For this review, take the finished solid that the model builds, in its own axes (mm). A direction names the side the tool comes from. Coordinates: 2 decimals unless noted, no trailing zeros. Write each loop counter-clockwise with the first axis right and the second up, starting at its lowest first coordinate (ties: lowest second). Pieces come first, ordered by that corner, then holes. Notation, with made-up numbers: (80.5, 22.25) -> (137.5, 22.25) arc R17 ccw to (137.5, 50.25) -> close; hole circle Ø4 at (-4.75, 87.25). An arc over 180 degrees is marked (long way). Put each result on its own line as item: value. Start each with the question number.
Item 1: To check wall thickness, follow L1, parallel to Y at x = 9, z = 0.15; L2, parallel to Y at x = -26.5, z = -1.75; L3, parallel to Y at x = 33, z = -1.2. State the ranges of each line that lie inside material, in increasing order.
Item 2: Consider section D-D on z = 0.15. Give the number of separate pieces and of enclosed holes in the cut face, and give its area (3 significant figures).
Item 3: Consider section B-B on x = 1. Give the boundary of the cut face in (y, z), and give its area (3 significant figures).
Item 4: Consider section C-C on y = 15. Give the boundary of the cut face in (x, z), and give its area (3 significant figures).
Item 5: For faces 4 (the flat face through (-20.334, -33.421, -1.44)), 5 (the flat face through (-35.9, 0, -2)), 6 (the flat face through (-7, 38, -0.7)), 7 (the flat face through (4.01, -24.66, 0.04)), 8 (the flat face through (35.9, 0, -2)), list the 3-axis set-ups (+Z, -Z, +X, -X, +Y, -Y) from which the entire face can be reached by the end or side of a thin tool; tool diameter is ignored.
Item 6: Consider section A-A on y = -7.5. Give the boundary of the cut face in (x, z).
Item 7: Insertion check: P1, Ø8, axis at x = 28, y = 39, coming from the -Z side; P2, Ø1.5, axis at y = -36.5, z = -1.5, coming from the +X side; P3, Ø1.1, axis at y = -6, z = -1.5, coming from the -X side. Each pin has a flat end and moves straight along its axis. Give the tip position at first contact, or say it passes through.
Item 8: The part is to be moulded in two halves that separate along Y. For faces 1 (the flat face through (20.7, -33.88, -1.44)), 2 (the flat face through (-1, 12, 0.8)), 3 (the flat face through (33.4, 14.8, -1.7)), say which applies: +Y half, -Y half, draft (parallel to the pull), parting line (faces both ways), or undercut.
```python
from build123d import *

# Parameters (mm, degrees)
ESBO_O2_W                = 80
ESBO_O2_H                = 100
ESBO_O2_W_2              = 55.6
ESBO_O2_H_2              = 18.4
RESSALTO_EXTRUS_O1_DEPTH = 0.8
RESSALTO_EXTRUS_O2_DEPTH = 2.2
CHANFRO3_SIZE            = 5
ESBO_O5_W                = 10
ESBO_O5_H                = 20
CORTE_EXTRUS_O1_DEPTH    = 10
CHANFRO4_SIZE            = 2
CHANFRO5_SIZE            = 2
RESSALTO_EXTRUS_O3_DEPTH = 0.7
ESBO_O7_W                = 61.8
ESBO_O7_H                = 24.6
ESBO_O7_W_2              = 55.6
ESBO_O7_H_2              = 18.4
RESSALTO_EXTRUS_O4_DEPTH = 2
ESBO_O8_W                = 61.8
ESBO_O8_H                = 24.6
RESSALTO_EXTRUS_O5_DEPTH = 0.6
CHANFRO6_SIZE            = 5
ESBO_O11_W               = 55.6
ESBO_O11_H               = 18.4
CORTE_EXTRUS_O2_DEPTH    = 0.9


with BuildPart() as part:
    # Esboço2 → Ressalto-extrusão1 (new body)
    with BuildSketch(Plane.XY):
        Rectangle(ESBO_O2_W, ESBO_O2_H)
        Rectangle(ESBO_O2_W_2, ESBO_O2_H_2, mode=Mode.SUBTRACT)
    extrude(amount=RESSALTO_EXTRUS_O1_DEPTH)

    # Esboço4 → Ressalto-extrusão2 (add)
    with BuildSketch(Plane(origin=(0, 0, 0), x_dir=(-1, 0, 0), z_dir=(0, 0, -1))):
        Polygon((40, -41.996094703), (20.243124237, -17.3), (35.9, -17.3), (35.9, 17.3), (20.243124237, 17.3), (40, 41.996094703), (40, 50), (33.596875763, 50), (7.436875763, 17.3), (-7.436875763, 17.3), (-33.596875763, 50), (-40, 50), (-40, 41.996094703), (-20.243124237, 17.3), (-35.9, 17.3), (-35.9, -17.3), (-20.243124237, -17.3), (-40, -41.996094703), (-40, -50), (-33.596875763, -50), (-7.436875763, -17.3), (7.436875763, -17.3), (33.596875763, -50), (40, -50), align=None)
        Polygon((3.436875763, 12.3), (5, 12.3), (16.243124237, 12.3), (30.9, 12.3), (30.9, -12.3), (16.243124237, -12.3), (5, -12.3), (3.436875763, -12.3), (-3.436875763, -12.3), (-5, -12.3), (-16.243124237, -12.3), (-30.9, -12.3), (-30.9, 12.3), (-16.243124237, 12.3), (-5, 12.3), (-2.810379517, 12.3), align=None, mode=Mode.SUBTRACT)
    extrude(amount=RESSALTO_EXTRUS_O2_DEPTH)

    # Chanfro3
    chanfro3_edges = [part.edges().sort_by_distance(p)[0] for p in [
        (-35.9, 17.3, -1.1),
        (35.9, 17.3, -1.1),
        (35.9, -17.3, -1.1),
        (-35.9, -17.3, -1.1),
    ]]
    chamfer(chanfro3_edges, length=CHANFRO3_SIZE)

    # Esboço5 → Corte-extrusão1 (cut)
    with BuildSketch(Plane(origin=(0, 0, 0), x_dir=(-1, 0, 0), z_dir=(0, 0, -1))):
        with Locations((0, 33.65)):
            Rectangle(ESBO_O5_W, ESBO_O5_H)
        with Locations((0, -33.65)):
            Rectangle(ESBO_O5_W, ESBO_O5_H)
    extrude(amount=-CORTE_EXTRUS_O1_DEPTH, mode=Mode.SUBTRACT)

    # Chanfro4
    chanfro4_edges = [part.edges().sort_by_distance(p)[0] for p in [
        (-5, 43.65, 0.4),
        (-5, 23.65, 0.4),
        (5, 23.65, 0.4),
        (5, 43.65, 0.4),
        (-5, -23.65, 0.4),
        (-5, -43.65, 0.4),
        (5, -43.65, 0.4),
        (5, -23.65, 0.4),
    ]]
    chamfer(chanfro4_edges, length=CHANFRO4_SIZE)

    # Chanfro5
    chanfro5_edges = [part.edges().sort_by_distance(p)[0] for p in [
        (-40, 50, -0.7),
        (40, 50, -0.7),
        (40, -50, -0.7),
        (-40, -50, -0.7),
    ]]
    chamfer(chanfro5_edges, length=CHANFRO5_SIZE)

    # Esboço6 → Ressalto-extrusão3 (add)
    # profile 1 of 4: a face of its own
    with BuildSketch(Plane(origin=(0, 0, 0), x_dir=(-1, 0, 0), z_dir=(0, 0, -1))):
        Polygon((30.9, -17.3), (20.243124237, -17.3), (40, -41.996094703), (40, 41.996094703), (20.243124237, 17.3), (30.9, 17.3), (35.9, 12.3), (35.9, -12.3), align=None)
    # profile 2 of 4: a face of its own
    with BuildSketch(Plane(origin=(0, 0, 0), x_dir=(-1, 0, 0), z_dir=(0, 0, -1))):
        Polygon((33.596875763, 50), (-33.596875763, 50), (-7.436875763, 17.3), (7.436875763, 17.3), align=None)
        Polygon((3, 43.65), (5, 41.65), (5, 25.65), (3, 23.65), (-3, 23.65), (-5, 25.65), (-5, 41.65), (-3, 43.65), align=None, mode=Mode.SUBTRACT)
    # profile 3 of 4: a face of its own
    with BuildSketch(Plane(origin=(0, 0, 0), x_dir=(-1, 0, 0), z_dir=(0, 0, -1))):
        Polygon((-40, -41.996094703), (-20.243124237, -17.3), (-30.9, -17.3), (-35.9, -12.3), (-35.9, 12.3), (-30.9, 17.3), (-20.243124237, 17.3), (-40, 41.996094703), align=None)
    # profile 4 of 4: a face of its own
    with BuildSketch(Plane(origin=(0, 0, 0), x_dir=(-1, 0, 0), z_dir=(0, 0, -1))):
        Polygon((33.596875763, -50), (7.436875763, -17.3), (-7.436875763, -17.3), (-33.596875763, -50), align=None)
        Polygon((-5, -25.65), (-5, -41.65), (-3, -43.65), (3, -43.65), (5, -41.65), (5, -25.65), (3, -23.65), (-3, -23.65), align=None, mode=Mode.SUBTRACT)
    extrude(amount=RESSALTO_EXTRUS_O3_DEPTH)

    # Esboço7 → Ressalto-extrusão4 (add)
    with BuildSketch(Plane(origin=(0, 0, 0), x_dir=(-1, 0, 0), z_dir=(0, 0, -1))):
        Rectangle(ESBO_O7_W, ESBO_O7_H)
        Rectangle(ESBO_O7_W_2, ESBO_O7_H_2, mode=Mode.SUBTRACT)
    extrude(amount=RESSALTO_EXTRUS_O4_DEPTH)

    # Esboço8 → Ressalto-extrusão5 (add)
    with BuildSketch(Plane(origin=(0, 0, -2.2), x_dir=(-1, 0, 0), z_dir=(0, 0, -1))):
        Polygon((30.9, 17.3), (-30.9, 17.3), (-35.9, 12.3), (-35.9, -12.3), (-30.9, -17.3), (30.9, -17.3), (35.9, -12.3), (35.9, 12.3), align=None)
        Rectangle(ESBO_O8_W, ESBO_O8_H, mode=Mode.SUBTRACT)
    extrude(amount=RESSALTO_EXTRUS_O5_DEPTH)

    # Chanfro6
    chanfro6_edges = [part.edges().sort_by_distance(p)[0] for p in [
        (-27.8, -9.2, -0.6),
        (27.8, -9.2, -0.6),
        (27.8, 9.2, -0.6),
        (-27.8, 9.2, -0.6),
    ]]
    chamfer(chanfro6_edges, length=CHANFRO6_SIZE)

    # Esboço11 → Corte-extrusão2 (cut)
    with BuildSketch(Plane(origin=(0, 0, -2), x_dir=(-1, 0, 0), z_dir=(0, 0, -1))):
        Rectangle(ESBO_O11_W, ESBO_O11_H)
    extrude(amount=-CORTE_EXTRUS_O2_DEPTH, mode=Mode.SUBTRACT)


solid = part.part
```
Return value:
1. L1: -50 to -9.2, 9.2 to 50
1. L2: -41.13 to -25.12, -17.3 to -9.2, 9.2 to 17.3, 25.12 to 41.13
1. L3: -49.25 to -33.25, -15.2 to 15.2, 33.25 to 49.25
2. separate pieces: 1
2. enclosed holes: 3
2. area: 6,630 mm^2
3. outline: (-50, -0.7) -> (-43.65, -0.7) -> (-43.65, 0.8) -> (-50, 0.8) -> close; (-23.65, -0.7) -> (-17.3, -0.7) -> (-17.3, -2.8) -> (-12.3, -2.8) -> (-12.3, -2) -> (-9.2, -2) -> (-9.2, 0.8) -> (-23.65, 0.8) -> close; (9.2, -2) -> (12.3, -2) -> (12.3, -2.8) -> (17.3, -2.8) -> (17.3, -0.7) -> (23.65, -0.7) -> (23.65, 0.8) -> (9.2, 0.8) -> close; (43.65, -0.7) -> (50, -0.7) -> (50, 0.8) -> (43.65, 0.8) -> close
3. area: 91.5 mm^2
4. outline: (-40, -0.7) -> (-33.2, -0.7) -> (-33.2, -2.8) -> (33.2, -2.8) -> (33.2, -0.7) -> (40, -0.7) -> (40, 0.8) -> (-40, 0.8) -> close
4. area: 259 mm^2
5. face 4: -Z, -Y
5. face 5: -Z, -X
5. face 6: -Z, +Y
5. face 7: +Z, -Z
5. face 8: -Z, +X
6. outline: (-40, -0.7) -> (-35.9, -0.7) -> (-35.9, -2.8) -> (-30.9, -2.8) -> (-30.9, -2) -> (-27.8, -2) -> (-27.8, -1.1) -> (-24.5, -1.1) -> (-24.5, 0.8) -> (-40, 0.8) -> close; (24.5, -1.1) -> (27.8, -1.1) -> (27.8, -2) -> (30.9, -2) -> (30.9, -2.8) -> (35.9, -2.8) -> (35.9, -0.7) -> (40, -0.7) -> (40, 0.8) -> (24.5, 0.8) -> close
7. P1: z = -2.2
7. P2: x = 36.2
7. P3: x = -35.9
8. face 1: -Y half
8. face 2: draft
8. face 3: undercut
